Geometry check sheet. Reference: the model listing, model coordinates, mm. A direction names the side the tool comes from. Round coordinates to 2 decimals unless told otherwise and drop trailing zeros. Write each loop counter-clockwise with the first axis right and the second up, starting at its lowest first coordinate (ties: lowest second). Pieces come first, ordered by that corner, then holes. Notation, with made-up numbers: M 40,-28 L 58,-28 A23 cw 58,9 Z; hole C 39,-26.75 d1. An arc over 180 degrees is marked long. One line per item, written item: value. Start each with the question number.
1. Access from +Z, -Z, +X, -X, +Y, -Y to the whole of each face (thin tool, end or side, straight path). Record for faces 1 (the cylindrical face through (7.843, 0.986, 7.804)), 2 (the cylindrical face through (21.715, 2.301, 0.21)), 3 (the cylindrical face through (-24.028, 5.934, 6.64)).
2. Section check C-C (x = 15.5). Record the boundary of the cut face in (y, z).
3. Depth check by flat-ended pin: P1, Ø2, axis at x = 6, z = -11.5, coming from the -Y side; P2, Ø8, axis at x = 0, z = 0, coming from the +Y side; P3, Ø12, axis at x = 10.5, z = 7, coming from the +Y side. Enter the tip coordinate at first touch or a pass-through.
4. Section check D-D (z = -2). Record the boundary of the cut face in (x, y).
5. Scan lines: probe 1 along Z at (x, y) = (6, 0.65); probe 2 along X at (y, z) = (5.5, 7.5); probe 3 along X at (y, z) = (0.95, 9). Record each from-to range of solid material in increasing order. Write a range as [from, to].
6. Section check A-A (y = 3.75). Record the boundary of the cut face in (x, z), and give its area (3 significant figures).
7. Section check B-B (z = 1.5). Record the boundary of the cut face in (x, y), and give its area (3 significant figures).
8. Release check for a two-part mould opening along Z. For faces 4 (the flat face through (-24.028, 10.072, 0.21)), 5 (the flat face through (5, 0, 0)), 6 (the cylindrical face through (-24.03, 6.07, -10.5)) record: pulls with the +Z half, pulls with the -Z half, needs draft (parallel to the pull), parting line crosses it, or undercut.
from build123d import *

# Parameters (mm, degrees)
ESBO_O1_W                = 52
ESBO_O1_H                = 30
ESBO_O1_R                = 4.5
ESBO_O1_R_2              = 1.205837633
RESSALTO_EXTRUS_O1_DEPTH = 2
ESBO_O2_R                = 1.5
RESSALTO_EXTRUS_O2_DEPTH = 4
FILETE3_R                = 1


with BuildPart() as part:
    # Esboço1 → Ressalto-extrusão1 (new body)
    with BuildSketch(Plane(origin=(0, 0, 0), x_dir=(1, 0, 0), z_dir=(0, 1, 0))):
        Rectangle(ESBO_O1_W, ESBO_O1_H)
        Circle(ESBO_O1_R, mode=Mode.SUBTRACT)
        with Locations((7, 7)):
            Circle(ESBO_O1_R_2, mode=Mode.SUBTRACT)
        with Locations((-6, 6)):
            Circle(ESBO_O1_R_2, mode=Mode.SUBTRACT)
        with Locations((-8, 9)):
            Circle(ESBO_O1_R_2, mode=Mode.SUBTRACT)
        with Locations((-7, -7)):
            Circle(ESBO_O1_R_2, mode=Mode.SUBTRACT)
        with Locations((6, -6)):
            Circle(ESBO_O1_R_2, mode=Mode.SUBTRACT)
        with Locations((8, -9)):
            Circle(ESBO_O1_R_2, mode=Mode.SUBTRACT)
    extrude(amount=RESSALTO_EXTRUS_O1_DEPTH)

    # Esboço2 → Ressalto-extrusão2 (add)
    with BuildSketch(Plane.ZY.offset(26)):
        Polygon((15, 2), (15, 12), (-15, 8.089445099), (-15, 2), align=None)
        with Locations((-9, 6)):
            Circle(ESBO_O2_R, mode=Mode.SUBTRACT)
        with BuildLine():
            ThreePointArc((8.240400933, 8.233448591), (9.539925295, 8.339457279), (10.431505763, 7.388097368))
            ThreePointArc((10.431505763, 7.388097368), (11.835840488, 7.245540316), (12.5, 6))
            ThreePointArc((12.5, 6), (11.226651005, 4.51722243), (9.568494237, 5.551902632))
            ThreePointArc((9.568494237, 5.551902632), (8.567535869, 5.503694052), (7.759599067, 6.096551409))
            ThreePointArc((7.759599067, 6.096551409), (6.624037685, 5.937880054), (5.708151293, 6.62768319))
            ThreePointArc((5.708151293, 6.62768319), (3.55555397, 8.354444888), (6.291848707, 8.71231681))
            ThreePointArc((6.291848707, 8.71231681), (7.357982, 8.84665675), (8.240400933, 8.233448591))
        make_face(mode=Mode.SUBTRACT)
    ressalto_extrus_o2 = extrude(amount=-RESSALTO_EXTRUS_O2_DEPTH)

    # Espelhar1: Ressalto-extrusão2 across plane
    add(ressalto_extrus_o2.mirror(Plane(origin=(0, 0, 0), x_dir=(0, 0, 1), z_dir=(1, 0, 0))))

    # Filete3
    filete3_edges = [part.edges().sort_by_distance(p)[0] for p in [
        (22, 2, 0),
        (-22, 2, 0),
    ]]
    fillet(filete3_edges, radius=FILETE3_R)


solid = part.part
Result sheet:
1. face 1: +Y, -Y
1. face 2: +Z, -Z, +Y
1. face 3: +X, -X
2. outline: M 0,-15 L 2,-15 L 2,15 L 0,15 Z
3. P1: stops at y = 0
3. P2: passes through
3. P3: stops at y = 2
4. outline: M -26,0 L -4.03,0 L -4.03,2 L -21,2 A1 cw -22,3 L -22,9.78 L -26,9.78 Z; M 4.03,0 L 26,0 L 26,9.78 L 22,9.78 L 22,3 A1 cw 21,2 L 4.03,2 Z
5. probe 1: z = [-15, -7.67], [-6.33, 4.79], [7.21, 15]
5. probe 2: x = [-26, -22], [22, 26]
5. probe 3: x = [-26, 6.79], [9.21, 26]
6. outline: M -26,-15 L -22,-15 L -22,15 L -26,15 Z; M 22,-15 L 26,-15 L 26,15 L 22,15 Z
6. area: 240 mm2
7. outline: M -26,0 L -4.24,0 L -4.24,2 L -21,2 A1 cw -22,3 L -22,10.24 L -26,10.24 Z; M 4.24,0 L 26,0 L 26,10.24 L 22,10.24 L 22,3 A1 cw 21,2 L 4.24,2 Z
7. area: 153 mm2
8. face 4: pulls with the -Z half
8. face 5: needs draft
8. face 6: undercut
